Autodesk Inventor part; units mm, degrees
ref_plane "YZ Plane" through (0, 0, 0) normal (1, 0, 0) x (0, 1, 0)
ref_plane "XZ Plane" through (0, 0, 0) normal (0, 1, 0) x (-1, 0, 0)
ref_plane "XY Plane" through (0, 0, 0) normal (0, 0, 1) x (1, 0, 0)
sketch "Sketch1" plane through (0, 0, 0) normal (0, 0, 1) x (1, 0, 0)
  line L0 (0, 0) -> (15, 0)
  line L1 (15, 0) -> (15, 12)
  line L2 (15, 12) -> (0, 12)
  line L3 (0, 12) -> (0, 0)
  line L4 (-7.5, 0) -> (22.5, 0)
  line L5 (22.5, 0) -> (22.5, -320)
  line L6 (-7.5, -320) -> (-7.5, 0)
  line L7 (0, -133) -> (15, -133)
  line L8 (15, -133) -> (15, -136)
  line L9 (15, -136) -> (0, -136)
  line L10 (0, -136) -> (0, -133)
  line L11 (15, -320) -> (15, -323)
  line L12 (15, -323) -> (0, -323)
  line L13 (0, -323) -> (0, -320)
  line L14 (22.5, -320) -> (15, -320)
  line L15 (0, -320) -> (-7.5, -320)
  line L16 (0, -223) -> (15, -223)
  line L17 (15, -223) -> (15, -226)
  line L18 (15, -226) -> (0, -226)
  line L19 (0, -226) -> (0, -223)
  point P0 (7.5, 12)
  point P1 (7.5, -320)
  point P2 (7.5, -133)
  point P3 (7.5, 0)
  point P4 (7.5, -323)
  point P5 (7.5, -223)
  dimension "d0" = 15
  dimension "d1" = 12
  dimension "d3" = 30
  dimension "d6" = 3
  dimension "d8" = 15
  dimension "d9" = 15
  dimension "d11" = 7.5
  dimension "d13" = 22.5
  dimension "d15" = 145
  dimension "d16" = 3
  dimension "d17" = 320
  dimension "d18" = 7.5
  dimension "d21" = 22.5
  dimension "d23" = 15
  dimension "d24" = 3
  dimension "d26" = 90
extrude "Extrusion1" add sketch "Sketch1" along normal blind 3
properties part number "back_down_hold"
Input: part model. Units: mm. Frame: model coordinates. Coordinates: 2 decimals unless noted, no trailing zeros. Order: outer loops, then holes, each group sorted by start corner. A loop starts at its lowest first (then second) coordinate and runs counter-clockwise, first axis right, second up.
1. Contact query for flat-ended pins moving along their axis: P1, Ø0.9, axis at x = 19.5, z = 2, coming from the -Y side; P2, Ø1.5, axis at y = -321, z = 1, coming from the +X side. Output: stop coordinate, or through.
Checked values:
P1: stops at y = -320
P2: stops at x = 15
2. Cut plane A-A, the plane x = 7. Return loops of the section in (y, z), plus the area to 3 significant figures.
Checked values:
outline: (-323, 0) - (-226, 0) - (-226, 3) - (-323, 3) - close; (-223, 0) - (-136, 0) - (-136, 3) - (-223, 3) - close; (-133, 0) - (12, 0) - (12, 3) - (-133, 3) - close
area: 987 mm2
3. Ray query, line 1 along Y through (x, z) = (4.5, 1.95); line 2 along Y through (x, z) = (19.5, 0.4). Return the intervals inside material, ascending.
Checked values:
line 1: y = -323 to -226, -223 to -136, -133 to 12
line 2: y = -320 to 0
4. Cut plane B-B, the plane z = 1.5. Return loops of the section in (x, y).
Checked values:
outline: (-7.5, -320) - (0, -320) - (0, -323) - (15, -323) - (15, -320) - (22.5, -320) - (22.5, 0) - (15, 0) - (15, 12) - (0, 12) - (0, 0) - (-7.5, 0) - close; hole (0, -226) - (15, -226) - (15, -223) - (0, -223) - close; hole (0, -136) - (15, -136) - (15, -133) - (0, -133) - close
